from build123d import *

# Parameters (mm, degrees)
BOSS_EXTRUDE1_DEPTH     = 10
CUT_EXTRUDE1_DEPTH      = 27.665192668
CUT_EXTRUDE1_DEPTH_BACK = 27.665192668
SKETCH2_R               = 2


with BuildPart() as part:
    # Sketch1 → Boss-Extrude1 (new body)
    with BuildSketch(Plane.XY):
        with BuildLine():
            Line((-7, 10.95445115), (-7, 8.614522622))
            ThreePointArc((-7, 8.614522622), (-9.855748076, 5.106293163), (-11.074633177, 0.75))
            Line((-11.074633177, 0.75), (-17.083544714, 0.75))
            ThreePointArc((-17.083544714, 0.75), (17.1, 0), (-17.083544714, -0.75))
            Line((-17.083544714, -0.75), (-11.074633177, -0.75))
            ThreePointArc((-11.074633177, -0.75), (-9.855748076, -5.106293163), (-7, -8.614522622))
            Line((-7, -8.614522622), (-7, -10.95445115))
            ThreePointArc((-7, -10.95445115), (0, -13), (7, -10.95445115))
            Line((7, -10.95445115), (7, -8.614522622))
            ThreePointArc((7, -8.614522622), (11.1, 0), (7, 8.614522622))
            Line((7, 8.614522622), (7, 10.95445115))
            ThreePointArc((7, 10.95445115), (0, 13), (-7, 10.95445115))
        make_face()
    extrude(amount=BOSS_EXTRUDE1_DEPTH)

    # Sketch2 → Cut-Extrude1 (cut, two sides: drawn at the far end of the back side and taken through both)
    with BuildSketch(Plane(origin=(0, -0.75, 0), x_dir=(1, 0, 0), z_dir=(0, 1, 0)).offset(-CUT_EXTRUDE1_DEPTH_BACK)):
        with Locations(Location((-14.079088945, -5, 0), (0, 0, 270))):
            Circle(SKETCH2_R)
    extrude(amount=CUT_EXTRUDE1_DEPTH + CUT_EXTRUDE1_DEPTH_BACK, mode=Mode.SUBTRACT)


solid = part.part
The model under review builds one solid part; all positions refer to its coordinate system, in mm. A direction names the side the tool comes from. Round coordinates to 2 decimals unless told otherwise and drop trailing zeros. Write each loop counter-clockwise with the first axis right and the second up, starting at its lowest first coordinate (ties: lowest second). Pieces come first, ordered by that corner, then holes. Notation, with made-up numbers: (31, 34.5) -> (81, 34.5) arc R26 ccw to (81, 53.5) -> close; hole circle Ø10 at (33, 34). An arc over 180 degrees is marked (long way). Answer as a JSON object with one key per item and string values.
1. To check wall thickness, follow line 1 along Y through (x, z) = (0.5, 4.5); line 2 along X through (y, z) = (-3.25, 5); line 3 along Y through (x, z) = (-8, 7.5). State the ranges of each line that lie inside material, in increasing order.
Results found:
{"line 1": "y = -17.09 to -12.99, 12.99 to 17.09", "line 2": "x = -16.79 to -16.08, -12.08 to -10.61, 10.61 to 16.79", "line 3": "y = -15.11 to -7.69, 7.69 to 15.11"}
2. We need section D-D on x = -4. State the section outline as (y, z) points, and give its area (3 significant figures).
Results found:
{"outline": "(-16.63, 0) -> (-12.37, 0) -> (-12.37, 10) -> (-16.63, 10) -> close; (12.37, 0) -> (16.63, 0) -> (16.63, 10) -> (12.37, 10) -> close", "area": "85.1 mm^2"}
3. Machinability: for faces 5 (the face through (-12.1, -5.2, 4.7)), 6 (the face through (-14.1, -0.75, 2.7)), 7 (the face through (-7, 10, 5)), which of the approach directions +Z, -Z, +X, -X, +Y, -Y give a long, thin tool a straight path to every point of the face, cutting with its end or side? Answer none if there is none.
Results found:
{"face 5": "+Y, -Y", "face 6": "+Z, -Z, -X", "face 7": "+Z, -Z"}
4. We need section A-A on x = 0. State the section outline as (y, z) points.
Results found:
{"outline": "(-17.1, 0) -> (-13, 0) -> (-13, 10) -> (-17.1, 10) -> close; (13, 0) -> (17.1, 0) -> (17.1, 10) -> (13, 10) -> close"}
5. We need section B-B on z = 2.25. State the section outline as (x, y) points, and give its area (3 significant figures).
Results found:
{"outline": "(-17.08, -0.75) arc R17.1 ccw (long way) to (-17.08, 0.75) -> (-11.07, 0.75) arc R11.1 cw to (-7, 8.61) -> (-7, 10.95) arc R13 cw to (7, 10.95) -> (7, 8.61) arc R11.1 cw to (7, -8.61) -> (7, -10.95) arc R13 cw to (-7, -10.95) -> (-7, -8.61) arc R11.1 cw to (-11.07, -0.75) -> close", "area": "466 mm^2"}
6. The part is to be moulded in two halves that separate along X. For faces 1 (the face through (17.084, 0.741, 4.93)), 2 (the face through (-9.885, -5.05, 4.93)), 3 (the face through (0, -13, 5)), 4 (the face through (-14, 0.75, 2.7)), say which applies: pulls with the +X half, pulls with the -X half, needs draft (parallel to the pull), parting line crosses it, or undercut.
Results found:
{"face 1": "parting line crosses it", "face 2": "undercut", "face 3": "undercut", "face 4": "needs draft"}
7. We need section C-C on z = 5. State the section outline as (x, y) points.
Results found:
{"outline": "(-17.08, -0.75) arc R17.1 ccw to (-16.08, -5.82) -> (-16.08, -0.75) -> close; (-17.08, 0.75) -> (-16.08, 0.75) -> (-16.08, 5.82) arc R17.1 ccw to start; (-12.08, -12.1) arc R17.1 ccw (long way) to (-12.08, 12.1) -> (-12.08, 0.75) -> (-11.07, 0.75) arc R11.1 cw to (-7, 8.61) -> (-7, 10.95) arc R13 cw to (7, 10.95) -> (7, 8.61) arc R11.1 cw to (7, -8.61) -> (7, -10.95) arc R13 cw to (-7, -10.95) -> (-7, -8.61) arc R11.1 cw to (-11.07, -0.75) -> (-12.08, -0.75) -> close"}
8. Clearance check with flat-ended pins moving along their axes: pin 1 (0.7 mm diameter, centred on y = 10, z = 5, fed in from -X); pin 2 (1.2 mm diameter, centred on y = -9.5, z = 3, fed in from -X); pin 3 (1 mm diameter, centred on x = 1.5, z = 5.5, fed in from -Y); pin 4 (2 mm diameter, centred on x = -2, y = 11, fed in from -Z). State where each tip first meets the part, or that it passes through.
Results found:
{"pin 1": "stops at x = -12.11", "pin 2": "stops at x = -14.6", "pin 3": "stops at y = -17.07", "pin 4": "passes through"}
